Study the drawing (mm; zero at the part's minimum x, y, z) and answer. Give positions to 0.01 mm unless a question says otherwise; leave off trailing zeros. Write each loop counter-clockwise with the first axis right and the second up, starting at its lowest first coordinate (ties: lowest second). Pieces come first, ordered by that corner, then holes.
1) Straight lines are drawn through the part: probe 1 along Y at (x, z) = (38, 3.5) (1 decimal); probe 2 along Y at (x, z) = (23.5, 3) (1 decimal); probe 3 along X at (y, z) = (28.5, 2.75). For each, find the intervals that lie inside material, in ascending order.
2) Determine the mould class of the marked faces 1, 2 and 3 for opening direction X: pulls with the +X half, pulls with the -X half, needs draft (parallel to the pull), parting line crosses it, or undercut.
3) Find section C-C (x = 40). Determine the outline of the cut face in (y, z) (1 decimal).
4) Find section A-A (x = 6). Determine the outline of the cut face in (y, z) (1 decimal).
5) Find section B-B (z = 5). Determine the outline of the cut face in (x, y) (1 decimal).
6) Given pin 1 Ø3 at (y, z) = (55.5, 4.5) entering from -X; pin 2 Ø3 at (y, z) = (55.5, 3) entering from +X; pin 3 Ø2 at (y, z) = (33.5, 1.5) entering from -X, each flat-ended and moving along its own axis, determine where each tip first touches the part or whether it passes through.
7) Find section D-D (y = 38). Determine the outline of the cut face in (x, z) (1 decimal).
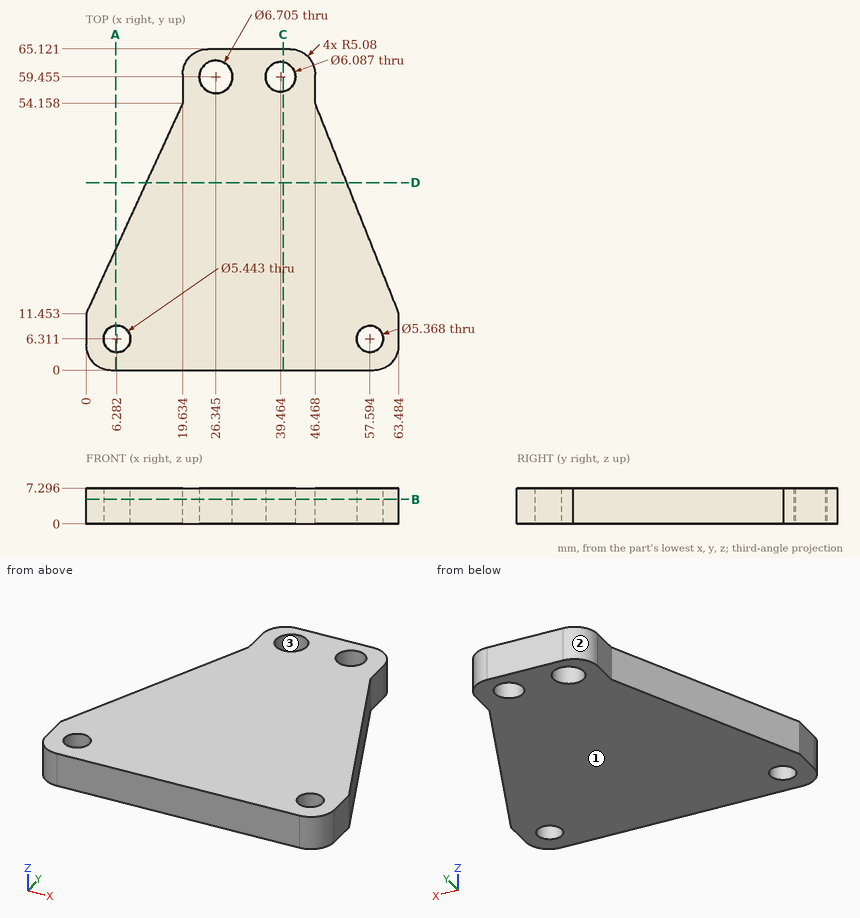
Results:
1. probe 1: y = 0 to 56.8, 62.1 to 65.1
1. probe 2: y = 0 to 57.7, 61.2 to 65
1. probe 3: x = 7.84 to 56.69
2. face 1: needs draft
2. face 2: pulls with the -X half
2. face 3: undercut
3. outline: (0, 0) - (56.5, 0) - (56.5, 7.3) - (0, 7.3) - close; (62.5, 0) - (65.1, 0) - (65.1, 7.3) - (62.5, 7.3) - close
4. outline: (0, 0) - (3.6, 0) - (3.6, 7.3) - (0, 7.3) - close; (9, 0) - (24.5, 0) - (24.5, 7.3) - (9, 7.3) - close
5. outline: (0, 5.1) arc R5.1 ccw to (5.1, 0) - (58.4, 0) arc R5.1 ccw to (63.5, 5.1) - (63.5, 11.5) - (46.5, 54.2) - (46.5, 60) arc R5.1 ccw to (41.4, 65.1) - (24.7, 65.1) arc R5.1 ccw to (19.6, 60) - (19.6, 54.2) - (0, 11.5) - close; hole circle Ø5.4 at (6.3, 6.3); hole circle Ø6.7 at (26.3, 59.5); hole circle Ø6.1 at (39.5, 59.5); hole circle Ø5.4 at (57.6, 6.3)
6. pin 1: stops at x = 19.56
6. pin 2: stops at x = 46.53
6. pin 3: stops at x = 9.68
7. outline: (12.2, 0) - (52.9, 0) - (52.9, 7.3) - (12.2, 7.3) - close
